For this review, take the finished solid that the model builds, in its own axes (mm). A direction names the side the tool comes from. Give positions to 0.01 mm unless a question says otherwise; leave off trailing zeros. Loops run counter-clockwise (first coordinate to the right, second up) from the corner with the lowest first, then second, coordinate; pieces in that order, holes last.
Autodesk Inventor part; units mm, degrees
ref_plane "YZ Plane" through (0, 0, 0) normal (1, 0, 0) x (0, 1, 0)
ref_plane "XZ Plane" through (0, 0, 0) normal (0, 1, 0) x (-1, 0, 0)
ref_plane "XY Plane" through (0, 0, 0) normal (0, 0, 1) x (1, 0, 0)
sketch "Sketch1" plane through (0, 0, 0) normal (0, 0, 1) x (1, 0, 0)
  circle A0 centre (0, 0.0481) radius 3
  circle A1 centre (0, 0.0481) radius 1.5
  circle A2 centre (0, 0.0481) radius 6.5
  arc A3 (2.6218, 17.0122) -> (-2.3779, 17.0481) centre (0.1221, 17.0481) ccw
  line L0 (0.1221, 17.0481) -> (-2.3779, 17.0481) construction
  line L1 (0.1221, 17.0481) -> (2.6221, 17.0481) construction
  line L2 (2.6221, 17.0481) -> (0.1221, 17.0481) construction
  line L3 (-2.3779, 17.0481) -> (-4.4642, 0.6149)
  line L4 (0.1221, 17.0481) -> (0, 0.0481) construction
  line L5 (2.6218, 17.0122) -> (4.4718, 0.5507)
  line L6 (0, 0.0481) -> (-9.4947, 0.1163) construction
  arc A4 (-2.6218, -16.916) -> (2.3779, -16.9519) centre (-0.1221, -16.9519) ccw
  line L7 (-2.6218, -16.916) -> (-4.4718, -0.4544)
  line L8 (2.3779, -16.9519) -> (4.4642, -0.5186)
  arc A5 (-4.4642, 0.6149) -> (-4.4718, -0.4544) centre (0, 0.0481) ccw
  arc A6 (4.4642, -0.5186) -> (4.4718, 0.5507) centre (0, 0.0481) ccw
  circle A7 centre (0, 0.0481) radius 4.5
  dimension "d1" = 3
  dimension "d2" = 6
  dimension "d4" = 13
  dimension "d5" = 5
  dimension "d6" = 17
  dimension "d8" = 16.5652
  dimension "d9" = 16.5652
  dimension "d10" = 97.235
  dimension "d20" = 13.9277
extrude "Extrusion1" add sketch "Sketch1" along normal blind 2 contours L5 A7 L3 A2 | A2 L3 A3 L5 | L8 A4 L7 A2 | A2 L7 A7 L8 | A6 A7 A5
extrude "Extrusion2" add sketch "Sketch1" along normal blind 2 contours A2 L8 A6 L5 | L5 A7 L3 A2 | A2 L7 A7 L8 | L3 A5 L7 A2 | A6 A7 A5
extrude "Extrusion3" add sketch "Sketch1" against normal blind 3.5 contours A6 A7 A5
extrude "Extrusion4" add sketch "Sketch1" along normal blind 1.75 contours A0
sketch "Sketch2" plane through (0, 0, 2) normal (0, 0, 1) x (1, 0, 0)
  circle A0 centre (0, 0.0481) radius 3
  circle A1 centre (0, 10.0481) radius 1.5
  circle A2 centre (0, -9.9519) radius 1.5
  dimension "d25" = 3
  dimension "d26" = 3
  dimension "d29" = 10
  dimension "d30" = 10
extrude "Extrusion5" cut sketch "Sketch2" against normal blind 2 contours A1 | A2
properties part number "acople estrella2 servo"
Item 1: The part is to be moulded in two halves that separate along X. For faces 6 (the cylindrical face through (-0.08, -19.45, 0.99)), 7 (the flat face through (1, -3, -3.5)), 8 (the cylindrical face through (-1.5, 0, 0.9)), say which applies: released by +X, released by -X, zero draft, split by the parting line, or undercut.
Answer:
face 6: split by the parting line
face 7: zero draft
face 8: undercut
Item 2: Take a section at B-B on z = 1.1. Give the boundary of the cut face in (x, y), and give its area (3 significant figures).
Answer:
outline: (-3.95, -5.12) - (-2.62, -16.92) arc R2.5 ccw (long way) to (2.38, -16.95) - (3.87, -5.17) arc R6.5 ccw to (3.95, 5.21) - (2.62, 17.01) arc R2.5 ccw (long way) to (-2.38, 17.05) - (-3.87, 5.27) arc R6.5 ccw to start; hole circle Ø3 at (0, -9.95); hole circle Ø3 at (0, 0.05); hole circle Ø3 at (0, 10.05)
area: 269 mm2
Item 3: For L1, parallel to Y at x = 0, z = 0.5; L2, parallel to Y at x = 0, z = 1.85; L3, parallel to Y at x = 0, z = -1.8, list the stretches that pass through material, from the lowest coordinate up.
Answer:
L1: y = -19.45 to -11.45, -8.45 to -1.45, 1.55 to 8.55, 11.55 to 19.55
L2: y = -19.45 to -11.45, -8.45 to -2.95, 3.05 to 8.55, 11.55 to 19.55
L3: y = -4.45 to -2.95, 3.05 to 4.55
Item 4: Clearance check with flat-ended pins moving along their axes: pin 1 Ø2 at (x, z) = (-0.5, -2.5) entering from -Y; pin 2 Ø1.5 at (y, z) = (7, 0.5) entering from -X; pin 3 Ø3 at (x, y) = (0.5, 0) entering from +Z; pin 4 Ø7 at (x, y) = (0, 0.05) entering from +Z. State where each tip first meets the part, or that it passes through.
Answer:
pin 1: stops at y = -4.45
pin 2: stops at x = -3.75
pin 3: stops at z = 1.75
pin 4: stops at z = 2
Item 5: Tool access review of faces 1 (the cylindrical face through (6.5, 0.1, 1)), 2 (the cylindrical face through (4.5, 0, -1.7)), 3 (the cylindrical face through (-6.5, 0, 1)), 4 (the flat face through (1.3, -1.2, 1.75)), 5 (the cylindrical face through (0.124, 4.546, -1.726)): name each direction out of +Z, -Z, +X, -X, +Y, -Y from which nothing blocks a thin tool from reaching the whole face with its end or side.
Answer:
face 1: +Z, -Z, +X
face 2: -Z, +X
face 3: +Z, -Z, -X
face 4: +Z
face 5: -Z, +Y
Item 6: Take a section at D-D on y = -6.5. Give the boundary of the cut face in (x, z).
Answer:
outline: (-3.79, 0) - (3.7, 0) - (3.7, 2) - (-3.79, 2) - close
Item 7: Take a section at C-C on z = -1.95. Give the boundary of the cut face in (x, y), and give its area (3 significant figures).
Answer:
outline: (-4.47, -0.45) arc R4.5 ccw to (4.46, -0.52) arc R4.5 ccw to (4.47, 0.55) arc R4.5 ccw to (-4.46, 0.61) arc R4.49 ccw to start; hole circle Ø6 at (0, 0.05)
area: 35.3 mm2
Item 8: Take a section at A-A on x = 0.25. Give the boundary of the cut face in (y, z), and give its area (3 significant figures).
Answer:
outline: (-19.42, 0) - (-11.43, 0) - (-11.43, 2) - (-19.42, 2) - close; (-8.47, 0) - (-4.44, 0) - (-4.44, -3.5) - (-2.94, -3.5) - (-2.94, 0) - (-1.43, 0) - (-1.43, 1.75) - (-2.94, 1.75) - (-2.94, 2) - (-8.47, 2) - close; (1.53, 0) - (3.04, 0) - (3.04, -3.5) - (4.54, -3.5) - (4.54, 0) - (8.57, 0) - (8.57, 2) - (3.04, 2) - (3.04, 1.75) - (1.53, 1.75) - close; (11.53, 0) - (19.54, 0) - (19.54, 2) - (11.53, 2) - close
area: 70.0 mm2
